Source: CAD feature listing. Evaluate the final solid. Frame: model axes, mm. Face numbers are marked on the shaded views. A direction names the side the tool comes from. Round coordinates to 2 decimals unless told otherwise and drop trailing zeros. Loops run counter-clockwise (first coordinate to the right, second up) from the corner with the lowest first, then second, coordinate; pieces in that order, holes last. Notation, with made-up numbers: (56, 89) - (105, 89) arc R18 ccw to (105, 121) - close; hole circle Ø8 at (77, -14). An arc over 180 degrees is marked (long way). One line per question, with ' | ' between items.
from build123d import *

# Parameters (mm, degrees)
SKETCH1_W                                           = 7.9375
SKETCH1_H                                           = 25.4
BOSS_EXTRUDE1_DEPTH                                 = 3.175
F_1_8_0_125_DIAMETER_HOLE1_D                        = 3.175
CBORE_FOR_2_BINDING_HEAD_MACHINE_SCREW1_D           = 2.4384
CBORE_FOR_2_BINDING_HEAD_MACHINE_SCREW1_CBORE_D     = 4.7625
CBORE_FOR_2_BINDING_HEAD_MACHINE_SCREW1_CBORE_DEPTH = 3.175
F_4_40_TAPPED_HOLE1_D                               = 2.2606
FILLET1_R                                           = 3.175
FILLET2_R                                           = 0.396875
CHAMFER2_SIZE                                       = 0.762
CHAMFER3_SIZE                                       = 0.254


with BuildPart() as part:
    # Sketch1 → Boss-Extrude1 (new body, symmetric)
    with BuildSketch(Plane.XY):
        Rectangle(SKETCH1_W, SKETCH1_H)
    extrude(amount=BOSS_EXTRUDE1_DEPTH, both=True)

    # 1/8 (0.125) Diameter Hole1 (through all)
    with Locations(Plane.XY.offset(3.175)):
        with Locations((0, 6.35)):
            Hole(F_1_8_0_125_DIAMETER_HOLE1_D / 2)

    # CBORE for #2 Binding Head Machine Screw1 (through all)
    with Locations(Plane.XY.offset(3.175)):
        with Locations((0, -1.5875), (0, -7.9375)):
            CounterBoreHole(CBORE_FOR_2_BINDING_HEAD_MACHINE_SCREW1_D / 2, CBORE_FOR_2_BINDING_HEAD_MACHINE_SCREW1_CBORE_D / 2, CBORE_FOR_2_BINDING_HEAD_MACHINE_SCREW1_CBORE_DEPTH)

    # #4-40 Tapped Hole1 (through all)
    with Locations(Plane.ZY.offset(3.96875)):
        with Locations((0, 6.35)):
            Hole(F_4_40_TAPPED_HOLE1_D / 2)

    # Fillet1
    fillet1_edges = [part.edges().sort_by_distance(p)[0] for p in [
        (-3.96875, -12.7, 0),
        (3.96875, -12.7, 0),
        (3.96875, 12.7, 0),
        (-3.96875, 12.7, 0),
    ]]
    fillet(fillet1_edges, radius=FILLET1_R)

    # Fillet2
    fillet2_edges = [part.edges().sort_by_distance(p)[0] for p in [
        (-2.38125, -7.9375, 0),
        (-2.38125, -1.5875, 0),
    ]]
    fillet(fillet2_edges, radius=FILLET2_R)

    # Chamfer2
    chamfer2_edges = [part.edges().sort_by_distance(p)[0] for p in [
        (0, 12.7, -3.175),
        (0, 12.7, 3.175),
        (-3.96875, 0, -3.175),
        (3.96875, 0, -3.175),
        (0, -12.7, -3.175),
        (-3.03881403, 11.77006403, -3.175),
        (-3.03881403, -11.77006403, -3.175),
        (3.03881403, -11.77006403, -3.175),
        (3.03881403, 11.77006403, -3.175),
        (3.96875, 0, 3.175),
        (-3.96875, 0, 3.175),
        (0, -12.7, 3.175),
        (-3.03881403, 11.77006403, 3.175),
        (-3.03881403, -11.77006403, 3.175),
        (3.03881403, -11.77006403, 3.175),
        (3.03881403, 11.77006403, 3.175),
    ]]
    chamfer(chamfer2_edges, length=CHAMFER2_SIZE)

    # Chamfer3
    chamfer3_edges = [part.edges().sort_by_distance(p)[0] for p in [
        (1.5875, 6.35, 3.175),
        (1.5875, 6.35, -3.175),
        (-2.38125, -7.9375, 3.175),
        (1.2192, -7.9375, -3.175),
        (1.2192, -7.9375, 0),
        (-2.38125, -1.5875, 3.175),
        (1.2192, -1.5875, -3.175),
        (1.2192, -1.5875, 0),
        (3.96875, 6.35, 1.1303),
        (-3.96875, 6.35, 1.1303),
    ]]
    chamfer(chamfer3_edges, length=CHAMFER3_SIZE)


solid = part.part
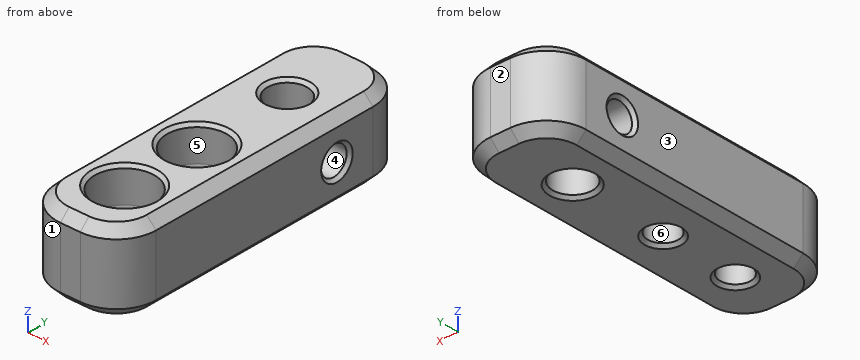
1. Section query A-A, the plane y = 3. Return loops of the section in (x, z) (3 decimals).
Worked out:
outline: (-3.969, -2.413) - (-3.207, -3.175) - (3.207, -3.175) - (3.969, -2.413) - (3.969, 2.413) - (3.207, 3.175) - (-3.207, 3.175) - (-3.969, 2.413) - close
2. Material intervals for probe 1 along Y at (x, z) = (0, 0.5); probe 2 along Z at (x, y) = (3.05, 6.35) (3 decimals); probe 3 along X at (y, z) = (6.35, 1.5), sorted ascending.
Worked out:
probe 1: y = -12.7 to -10.32, -5.56 to -3.97, 0.79 to 4.76, 7.94 to 12.7 | probe 2: z = -3.175 to -1.13, 1.13 to 3.175 | probe 3: x = -3.97 to -1.59, 1.59 to 3.97
3. Access query for the marked faces 5 and 6. Directions: +Z, -Z, +X, -X, +Y, -Y. A direction counts if a zero-diameter tool reaches every point of the face in a straight line with its end or side. Return the directions, or none.
Worked out:
face 5: +Z | face 6: +Z, -Z
4. Contact query for flat-ended pins moving along their axis: P1, Ø3, axis at x = 0, y = -7.94, coming from the +Z side; P2, Ø3, axis at x = 0, y = 6.35, coming from the -Z side; P3, Ø2.5, axis at y = 6.35, z = 0, coming from the +X side. Output: stop coordinate, or through.
Worked out:
P1: stops at z = 0 | P2: passes through | P3: stops at x = 3.83
5. Mould query, pull axis Y, two halves, no side actions, for the marked faces 1, 2, 3 and 4. Classes: released by +Y, released by -Y, zero draft, split by the parting line, or undercut.
Worked out:
face 1: released by -Y | face 2: released by +Y | face 3: zero draft | face 4: undercut
6. Section query B-B, the plane y = 6.35. Give the number of separate pieces and of enclosed holes in the cut face, plus the area to 3 significant figures.
Worked out:
separate pieces: 4 | enclosed holes: 0 | area: 18.1 mm2
